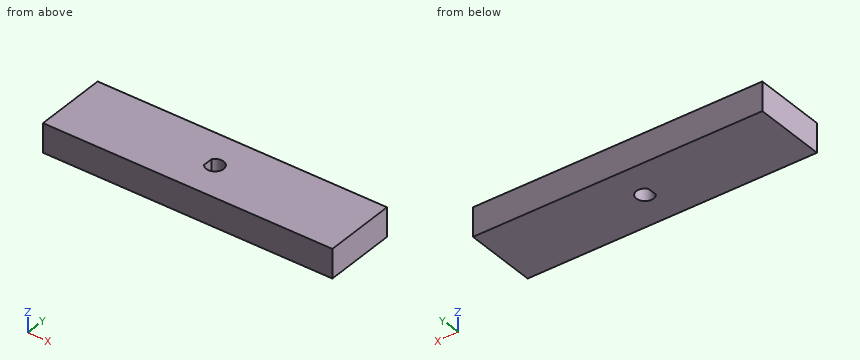
from build123d import *

# Parameters (mm, degrees)
SKETCH1_W           = 100
SKETCH1_H           = 25
BOSS_EXTRUDE1_DEPTH = 10
CUT_EXTRUDE1_DEPTH  = 10


with BuildPart() as part:
    # Sketch1 → Boss-Extrude1 (new body)
    with BuildSketch(Plane.XY):
        Rectangle(SKETCH1_W, SKETCH1_H)
    extrude(amount=BOSS_EXTRUDE1_DEPTH)

    # Sketch2 → Cut-Extrude1 (cut)
    with BuildSketch(Plane.XY.offset(10)):
        with BuildLine():
            Line((-2.5, 1.658312395), (-2.5, -1.658312395))
            ThreePointArc((-2.5, -1.658312395), (3, 0), (-2.5, 1.658312395))
        make_face()
    extrude(amount=-CUT_EXTRUDE1_DEPTH, mode=Mode.SUBTRACT)


solid = part.part
Model file for the job. Use its own axes, mm. Coordinates: 2 decimals unless noted, no trailing zeros. Write each loop counter-clockwise with the first axis right and the second up, starting at its lowest first coordinate (ties: lowest second). Pieces come first, ordered by that corner, then holes. Notation, with made-up numbers: (34, 82) - (68, 82) arc R18 ccw to (68, 102) - close; hole circle Ø4 at (-21, 16.25). An arc over 180 degrees is marked (long way). Write each question's results on one line, items separated by ' | '. Start each with the question number.
1) Cut at A-A (y = 0). Write the cut outline in (x, z).
2) Probe line 1 along X through (y, z) = (0, 7.75); line 2 along Y through (x, z) = (0, 7); line 3 along X through (y, z) = (2.25, 3.75). List the from-to ranges inside material, lowest first. Write a range as from..to.
3) Cut at B-B (x = 0). Write the cut outline in (y, z).
4) Flat gauge pin, fed straight in: P1, Ø6, axis at x = 34.5, y = -2.5, coming from the -Z side. Where does the tip first touch, or does it go through?
Returned:
1) outline: (-50, 0) - (-2.5, 0) - (-2.5, 10) - (-50, 10) - close; (3, 0) - (50, 0) - (50, 10) - (3, 10) - close
2) line 1: -50..-2.5, 3..50 | line 2: -12.5..-3, 3..12.5 | line 3: -50..-1.98, 1.98..50
3) outline: (-12.5, 0) - (-3, 0) - (-3, 10) - (-12.5, 10) - close; (3, 0) - (12.5, 0) - (12.5, 10) - (3, 10) - close
4) P1: z = 0
